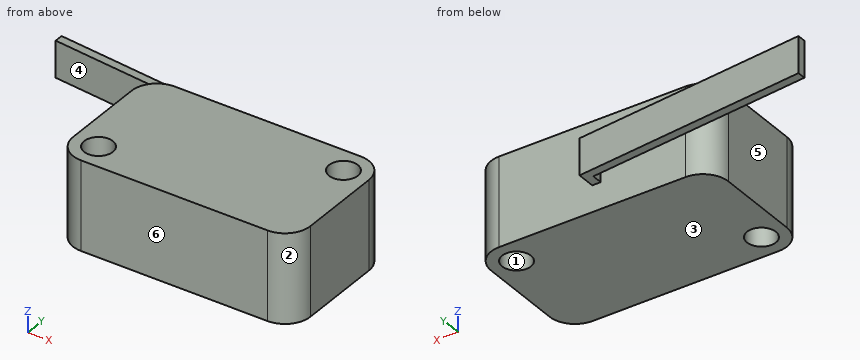
```python
from build123d import *

# Parameters (mm, degrees)
SKETCH_1_W          = 28
SKETCH_1_H          = 16
EXTRUDE_1_DEPTH     = 10.5
SKETCH_2_R          = 1.7
CUT_EXTRUDE_1_DEPTH = 10.5
FILLET_1_R          = 3
EXTRUDE_2_DEPTH     = 10.5
SKETCH_4_W          = 27.845387087
SKETCH_4_H          = 5.10555255
CUT_EXTRUDE_2_DEPTH = 3.1
SKETCH_5_W          = 33.643456051
SKETCH_5_H          = 7.59321446
CUT_EXTRUDE_3_DEPTH = 3.1


with BuildPart() as part:
    # 草图1 → 凸台-拉伸1 (new body)
    with BuildSketch(Plane.XY):
        Rectangle(SKETCH_1_W, SKETCH_1_H)
    extrude(amount=EXTRUDE_1_DEPTH)

    # 草图2 → 切除-拉伸1 (cut)
    with BuildSketch(Plane.XY.offset(10.5)):
        with Locations((-11, -5)):
            Circle(SKETCH_2_R)
        with Locations((11, 5)):
            Circle(SKETCH_2_R)
    extrude(amount=-CUT_EXTRUDE_1_DEPTH, mode=Mode.SUBTRACT)

    # 圆角1
    fillet_1_edges = [part.edges().sort_by_distance(p)[0] for p in [
        (-14, 8, 5.25),
        (14, 8, 5.25),
        (14, -8, 5.25),
        (-14, -8, 5.25),
    ]]
    fillet(fillet_1_edges, radius=FILLET_1_R)

    # 草图3 → 凸台-拉伸2 (add)
    with BuildSketch(Plane.XY):
        Polygon((0, 8), (0, 10.167114537), (-27.845387087, 13.10555255), (-27.845387087, 12.1), (-1, 9.267088909), (-1, 8), align=None)
    extrude(amount=EXTRUDE_2_DEPTH)

    # 草图4 → 切除-拉伸2 (cut)
    with BuildSketch(Plane.XY.offset(10.5)):
        with Locations((-13.922693544, 10.552776275)):
            Rectangle(SKETCH_4_W, SKETCH_4_H)
    extrude(amount=-CUT_EXTRUDE_2_DEPTH, mode=Mode.SUBTRACT)

    # 草图5 → 切除-拉伸3 (cut)
    with BuildSketch(Plane(origin=(0, 0, 0), x_dir=(-1, 0, 0), z_dir=(0, 0, -1))):
        with Locations((16.821728026, 11.79660723)):
            Rectangle(SKETCH_5_W, SKETCH_5_H)
    extrude(amount=-CUT_EXTRUDE_3_DEPTH, mode=Mode.SUBTRACT)


solid = part.part
```
Part model, mm, in its own coordinate system. Face numbers are marked on the shaded views. A direction names the side the tool comes from. Round coordinates to 2 decimals unless told otherwise and drop trailing zeros. Write each loop counter-clockwise with the first axis right and the second up, starting at its lowest first coordinate (ties: lowest second). Pieces come first, ordered by that corner, then holes. Notation, with made-up numbers: M 47,79.25 L 68,79.25 A25 ccw 68,105.25 Z; hole C 27,-40 d8. An arc over 180 degrees is marked long. Answer as CSV lines item,"result". Start each with the question number.
1) Band-saw the part on D-D (x = 3.5). List the corners of the cut face in (y, z), then the cut area to 3 significant figures.
2) Drop flat-ended pins along their axis: pin 1 (5 mm diameter, centred on x = -2, z = 5, fed in from +Y); pin 2 (0.7 mm diameter, centred on y = 9, z = 5.5, fed in from +X); pin 3 (4.5 mm diameter, centred on x = 11, y = 5, fed in from +Z); pin 4 (5 mm diameter, centred on x = -21, z = 4.5, fed in from +Y). Give the stop position or say it passes through.
3) Band-saw the part on A-A (z = 3.5). List the corners of the cut face in (x, y), then the cut area to 3 significant figures.
4) Which spindle directions (+Z, -Z, +X, -X, +Y, -Y) get a long thin tool onto all of the face, cutting with end or side? Do the marked faces 4, 5 and 6. Say none if no direction does.
5) Drill centre lines: L1, parallel to Y at x = 11, z = 3.75; L2, parallel to Y at x = -11, z = 2.75; L3, parallel to X at y = -0.75, z = 2.25. Where is each one in solid material? Low to high.
6) Band-saw the part on C-C (y = 8.75). List the corners of the cut face in (x, z), then the cut area to 3 significant figures.
7) Band-saw the part on B-B (x = -10). List the corners of the cut face in (y, z).
8) Mould opens along X. For the marked faces 1, 2 and 3 say: +X half, -X half, draft (parallel to the pull), parting line (faces both ways), or undercut.
Worked out:
1,outline,"M -8,0 L 8,0 L 8,10.5 L -8,10.5 Z"
1,area,"168 mm²"
2,pin 1,"y = 10.64"
2,pin 2,"x = 0"
2,pin 3,"z = 10.5"
2,pin 4,"y = 12.65"
3,outline,"M -27.85,12.1 L -1,9.27 L -1,8 L -11,8 A3 ccw -14,5 L -14,-5 A3 ccw -11,-8 L 11,-8 A3 ccw 14,-5 L 14,5 A3 ccw 11,8 L 0,8 L 0,10.17 L -27.85,13.11 Z; hole C -11,-5 d3.4; hole C 11,5 d3.4"
3,area,"451 mm²"
4,face 4,"+Z, -Z, -X"
4,face 5,"+Z, -Z, -X, -Y"
4,face 6,"+Z, -Z, +X, -X, -Y"
5,L1,"-8 to 3.3, 6.7 to 8"
5,L2,"-8 to -6.7, -3.3 to 8"
5,L3,"-14 to 14"
6,outline,"M -1,3.1 L 0,3.1 L 0,7.4 L -1,7.4 Z"
6,area,"4.30 mm²"
7,outline,"M -8,0 L -6.37,0 L -6.37,10.5 L -8,10.5 Z; M -3.63,0 L 8,0 L 8,10.5 L -3.63,10.5 Z; M 10.22,3.1 L 11.22,3.1 L 11.22,7.4 L 10.22,7.4 Z"
8,face 1,"undercut"
8,face 2,"+X half"
8,face 3,"draft"
